```python
from build123d import *

# Parameters (mm, degrees)
F0_R     = 5.08
F0_W     = 10.16
F0_H     = 15.24
F1_DEPTH = 3.81
F2_W     = 13.9550012536
F2_H     = 12.9558886401
F3_DEPTH = 12.7
F4_R     = 5.08
F5_DEPTH = 3.81


with BuildPart() as f1:
    # F0 (on Top) → F1 (new body)
    with BuildSketch(Plane.XY):
        with BuildLine():
            Line((17.78, 7.5147451945), (-17.78, 7.5147451945))
            ThreePointArc((-17.78, 7.5147451945), (-25.4, -0.1052548055), (-17.78, -7.7252548055))
            Line((-17.78, -7.7252548055), (-11.43, -7.7252548055))
            Line((-11.43, -7.7252548055), (-5.08, -7.7252548055))
            Line((-5.08, -7.7252548055), (0, -7.7252548055))
            Line((0, -7.7252548055), (5.08, -7.7252548055))
            Line((5.08, -7.7252548055), (11.43, -7.7252548055))
            Line((11.43, -7.7252548055), (17.78, -7.7252548055))
            ThreePointArc((17.78, -7.7252548055), (25.4, -0.1052548055), (17.78, 7.5147451945))
        make_face()
        with Locations((-17.78, -0.1052548055)):
            Circle(F0_R, mode=Mode.SUBTRACT)
        with Locations((17.78, -0.1052548055)):
            Circle(F0_R, mode=Mode.SUBTRACT)
        Polygon((-5.08, -7.7252548055), (-11.43, -7.7252548055), (-5.08, -17.8852548055), align=None)
        Polygon((5.08, -17.8852548055), (11.43, -7.7252548055), (5.08, -7.7252548055), align=None)
        Polygon((0, -7.7252548055), (-5.08, -7.7252548055), (-5.08, -17.8852548055), (5.08, -17.8852548055), (5.08, -7.7252548055), align=None)
        with Locations((0, -25.5052548055)):
            Rectangle(F0_W, F0_H)
    extrude(amount=F1_DEPTH)

    # F2 (on face) → F3 (join)
    with BuildSketch(Plane.XY.offset(3.81)):
        with Locations((0.3611810971, -0.169222476)):
            Rectangle(F2_W, F2_H)
    extrude(amount=F3_DEPTH)

    # F4 (on face) → F5 (join)
    with BuildSketch(Plane.XY.offset(16.51)):
        with BuildLine():
            Line((17.78, 7.5147451945), (-17.78, 7.5147451945))
            ThreePointArc((-17.78, 7.5147451945), (-25.4, -0.1052548055), (-17.78, -7.7252548055))
            Line((-17.78, -7.7252548055), (-11.43, -7.7252548055))
            Line((-11.43, -7.7252548055), (11.43, -7.7252548055))
            Line((11.43, -7.7252548055), (17.78, -7.7252548055))
            ThreePointArc((17.78, -7.7252548055), (25.4, -0.1052548055), (17.78, 7.5147451945))
        make_face()
        with Locations((-17.78, -0.1052548055)):
            Circle(F4_R, mode=Mode.SUBTRACT)
        with Locations((17.78, -0.1052548055)):
            Circle(F4_R, mode=Mode.SUBTRACT)
    extrude(amount=F5_DEPTH)


solid = f1.part
```
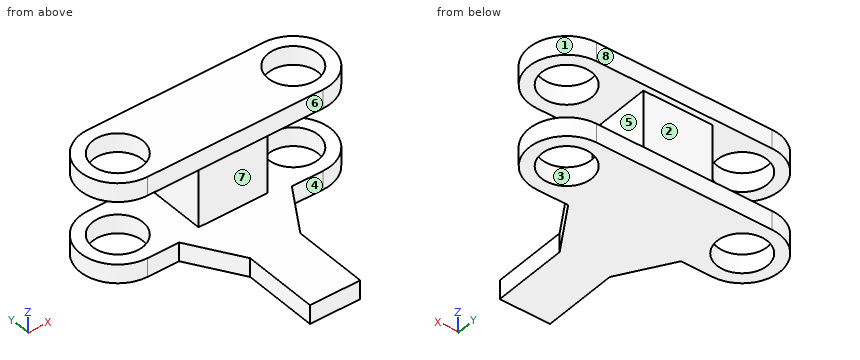
Geometry check sheet. Reference: the model listing, model coordinates, mm. Face numbers are marked on the shaded views. A direction names the side the tool comes from. Round coordinates to 2 decimals unless told otherwise and drop trailing zeros. Loops run counter-clockwise (first coordinate to the right, second up) from the corner with the lowest first, then second, coordinate; pieces in that order, holes last. Notation, with made-up numbers: (12.25, 58) - (50.25, 58) arc R20 ccw to (50.25, 68) - close; hole circle Ø8 at (85.5, 83). An arc over 180 degrees is marked (long way). Use a Markdown table: item, result.
Q1. Cross-section at A-A on x = -8. Record the cut outline in (y, z).
Solutions:
| item | result |
|---|---|
| outline | (-13.21, 0) - (7.51, 0) - (7.51, 3.81) - (-13.21, 3.81) - close; (-7.73, 16.51) - (7.51, 16.51) - (7.51, 20.32) - (-7.73, 20.32) - close |
Q2. Cross-section at B-B on z = 3. Record the cut outline in (x, y).
Solutions:
| item | result |
|---|---|
| outline | (-17.78, -7.73) - (-11.43, -7.73) - (-5.08, -17.89) - (-5.08, -33.13) - (5.08, -33.13) - (5.08, -17.89) - (11.43, -7.73) - (17.78, -7.73) arc R7.62 ccw to (17.78, 7.51) - (-17.78, 7.51) arc R7.62 ccw to start; hole circle Ø10.16 at (-17.78, -0.11); hole circle Ø10.16 at (17.78, -0.11) |
Q3. Go/stop test with flat-tipped pins: P1, Ø10, axis at x = -12.5, y = -28.5, coming from the +Z side; P2, Ø13, axis at x = -17.78, y = -0.11, coming from the -Z side; P3, Ø4, axis at y = -2.5, z = 10, coming from the +X side; P4, Ø3, axis at x = 16, z = 2.5, coming from the -Y side. Record where each tip stops, or that it passes through.
Solutions:
| item | result |
|---|---|
| P1 | passes through |
| P2 | stops at z = 0 |
| P3 | stops at x = 7.34 |
| P4 | stops at y = -7.73 |
Q4. Material ranges on line 1 (Y direction, x = -17.78, z = 18.25); line 2 (Z direction, x = 12, y = 5); line 3 (X direction, y = -27, z = 1), recorded low to high.
Solutions:
| item | result |
|---|---|
| line 1 | y = -7.73 to -5.19, 4.97 to 7.51 |
| line 2 | z = 0 to 3.81, 16.51 to 20.32 |
| line 3 | x = -5.08 to 5.08 |
Q5. Draft check along Y on the marked faces 1, 2 and 3. Enter one of: released by +Y, released by -Y, zero draft, split by the parting line, or undercut.
Solutions:
| item | result |
|---|---|
| face 1 | split by the parting line |
| face 2 | released by +Y |
| face 3 | undercut |
Q6. Access from +Z, -Z, +X, -X, +Y, -Y to the whole of each face (thin tool, end or side, straight path). Record for the marked faces 4, 5, 6, 7 and 8.
Solutions:
| item | result |
|---|---|
| face 4 | +Z, -Z, +X, -Y |
| face 5 | +X, +Y, -Y |
| face 6 | +Z, +X, -X, -Y |
| face 7 | +X, -X, -Y |
| face 8 | +Z, -Z, +X, -X, +Y |
Q7. Cross-section at D-D on y = -4.5. Record the cut outline in (x, z) (3 decimals).
Solutions:
| item | result |
|---|---|
| outline | (-24.005, 0) - (-20.328, 0) - (-20.328, 3.81) - (-24.005, 3.81) - close; (-24.005, 16.51) - (-20.328, 16.51) - (-20.328, 20.32) - (-24.005, 20.32) - close; (-15.232, 0) - (15.232, 0) - (15.232, 3.81) - (7.339, 3.81) - (7.339, 16.51) - (15.232, 16.51) - (15.232, 20.32) - (-15.232, 20.32) - (-15.232, 16.51) - (-6.616, 16.51) - (-6.616, 3.81) - (-15.232, 3.81) - close; (20.328, 0) - (24.005, 0) - (24.005, 3.81) - (20.328, 3.81) - close; (20.328, 16.51) - (24.005, 16.51) - (24.005, 20.32) - (20.328, 20.32) - close |
Q8. Cross-section at C-C on x = 2. Record the cut outline in (y, z).
Solutions:
| item | result |
|---|---|
| outline | (-33.13, 0) - (7.51, 0) - (7.51, 3.81) - (6.31, 3.81) - (6.31, 16.51) - (7.51, 16.51) - (7.51, 20.32) - (-7.73, 20.32) - (-7.73, 16.51) - (-6.65, 16.51) - (-6.65, 3.81) - (-33.13, 3.81) - close |
